Could you check a few things on this model? Use its own coordinates, in mm. Face numbers are marked on the shaded views. A direction names the side the tool comes from. Round coordinates to 2 decimals unless told otherwise and drop trailing zeros. Order: outer loops, then holes, each group sorted by start corner. A loop starts at its lowest first (then second) coordinate and runs counter-clockwise, first axis right, second up. Notation, with made-up numbers: (-21, 35.25) -> (-10, 35.25) arc R30 cw to (-10, 60.25) -> close; hole circle Ø5 at (43, -36.75). An arc over 180 degrees is marked (long way). One line per question, with ' | ' between items.
```python
from build123d import *

# Parameters (mm, degrees)
F0_W     = 2
F0_H     = 3
F1_DEPTH = 8


with BuildPart() as f1:
    # F0 (on Top) → F1 (new body)
    with BuildSketch(Plane.XY):
        with BuildLine():
            ThreePointArc((24.046684, 38.003651), (17.604921, 41.125799), (10.5, 42))
            ThreePointArc((10.5, 42), (15.717908, 40.668619), (19.660035, 37))
            Line((19.660035, 37), (24.046684, 38.003651))
        make_face()
        with BuildLine():
            ThreePointArc((10.5, 42), (3.899811, 39.772124), (0, 34))
            Line((0, 34), (3.2, 34))
            ThreePointArc((3.2, 34), (9.6069, 38.747985), (16.933573, 35.599717))
            ThreePointArc((16.933573, 35.599717), (17.027709, 34.552628), (16.133361, 34))
            Line((16.133361, 34), (15, 34))
            Line((15, 34), (15, 32))
            Line((15, 32), (20, 32))
            ThreePointArc((20, 32), (20.707107, 32.292893), (21, 33))
            Line((21, 33), (21, 34))
            ThreePointArc((21, 34), (20.443805, 35.550823), (19.660035, 37))
            ThreePointArc((19.660035, 37), (15.717908, 40.668619), (10.5, 42))
        make_face()
        with Locations((4.2, 1.5)):
            Rectangle(F0_W, F0_H)
        with BuildLine():
            ThreePointArc((0, 1), (0.292893, 0.292893), (1, 0))
            Line((1, 0), (3.2, 0))
            Line((3.2, 0), (3.2, 3))
            Line((3.2, 3), (3.2, 34))
            Line((3.2, 34), (0, 34))
            Line((0, 34), (0, 1))
        make_face()
    extrude(amount=F1_DEPTH)


solid = f1.part
```
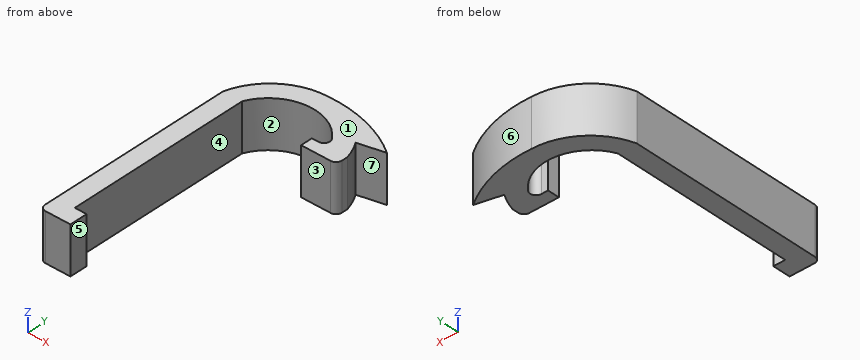
1. I need wall thicknesses on probe 1 along X at (y, z) = (35.5, 2.25); probe 2 along X at (y, z) = (34.5, 2.75); probe 3 along X at (y, z) = (18.5, 3.5). Which ranges of each line are inside material? Lowest first, please.
From the geometry:
probe 1: x = 0.53 to 4.06, 17 to 20.47 | probe 2: x = 0.15 to 3.44, 17 to 20.85 | probe 3: x = 0 to 3.2
2. I want a section at A-A on x = 4.25. List the corners of the cut face in (y, z) for me, and give its area (3 significant figures).
From the geometry:
outline: (0, 0) -> (3, 0) -> (3, 8) -> (0, 8) -> close; (35.75, 0) -> (40.03, 0) -> (40.03, 8) -> (35.75, 8) -> close | area: 58.2 mm²
3. I'm going to push flat-ended pins straight in: pin 1 (3 mm diameter, centred on y = 37.5, z = 5.5, fed in from -X); pin 2 (2 mm diameter, centred on y = 33, z = 5.5, fed in from -X); pin 3 (1.5 mm diameter, centred on x = 17, z = 3.5, fed in from -Y); pin 4 (0.6 mm diameter, centred on x = 4, z = 3.5, fed in from +Y). Where does each tip first touch, or does it pass through?
From the geometry:
pin 1: stops at x = 0.77 | pin 2: stops at x = 0 | pin 3: stops at y = 32 | pin 4: stops at y = 40.06
4. If we mould it in two halves opening along Y, with no side actions, what happens to the marked faces 4, 5, 6 and 7? For each: pulls with the +Y half, pulls with the -Y half, needs draft (parallel to the pull), parting line crosses it, or undercut.
From the geometry:
face 4: undercut | face 5: needs draft | face 6: pulls with the +Y half | face 7: undercut
5. On a 3-axis mill with a long thin cutter (end or side, diameter ignored), from which of +Z, -Z, +X, -X, +Y, -Y can I reach the whole of each face in a straight line? I mean the marked faces 1, 2 and 3. Say none if no direction works.
From the geometry:
face 1: +Z, +X, -X, +Y, -Y | face 2: +Z, -Z | face 3: +Z, -Z, +X, -Y
6. I want a section at D-D on x = 14.5. List the corners of the cut face in (y, z) for me.
From the geometry:
outline: (37.75, 0) -> (41.8, 0) -> (41.8, 8) -> (37.75, 8) -> close
7. I want a section at B-B on z = 6.5. List the corners of the cut face in (x, y) for me, and give its area (3 significant figures).
From the geometry:
outline: (0, 1) arc R1 ccw to (1, 0) -> (5.2, 0) -> (5.2, 3) -> (3.2, 3) -> (3.2, 34) arc R8 cw to (16.93, 35.6) arc R1 cw to (16.13, 34) -> (15, 34) -> (15, 32) -> (20, 32) arc R1 ccw to (21, 33) -> (21, 34) arc R10.89 ccw to (19.66, 37) -> (24.05, 38) arc R21.86 ccw to (10.5, 42) arc R10.89 ccw to (0, 34) -> close | area: 218 mm²
8. I want a section at C-C on y = 26.5. List the corners of the cut face in (x, z) for me, and give its area (3 significant figures).
From the geometry:
outline: (0, 0) -> (3.2, 0) -> (3.2, 8) -> (0, 8) -> close | area: 25.6 mm²
